Geometry: final body of the model. Coordinates: model frame, mm. Give positions to 0.01 mm unless a question says otherwise; leave off trailing zeros. Write each loop counter-clockwise with the first axis right and the second up, starting at its lowest first coordinate (ties: lowest second). Pieces come first, ordered by that corner, then holes. Notation, with made-up numbers: M 87,-10.5 L 121,-10.5 A24 ccw 121,28.5 Z; hole C 4,-19 d6. An arc over 180 degrees is marked long. Use a Markdown table: item, result. Add a question column.
(1) Cut plane C-C (x = 26.6). State how many separate pieces and enclosed holes the cut face has, plus the area to 3 significant figures.
(2) Pin query (flat end, axial travel): pin 1 Ø5 at (y, z) = (1, -15.5) entering from -X; pin 2 Ø12 at (x, z) = (-31, 3.5) entering from +Y; pin 3 Ø3.5 at (x, z) = (4.2, 10.4) entering from -Y. Return the tip coordinate at first contact, or that it passes through.
(3) Cut plane B-B (z = -17.5). Output: boundary loops of the cut face in (x, y), plus the area to 3 significant figures.
(4) Cut plane A-A (x = -168). Output: boundary loops of the cut face in (y, z), plus the area to 3 significant figures.
(5) Material intervals for L1, parallel to Y at x = -2, z = -4.5; L2, parallel to Z at x = -153, y = 3.5, sorted ascending.
```python
from build123d import *

# Parameters (mm, degrees)
SKETCH1_R           = 3
BOSS_EXTRUDE2_DEPTH = 5
SKETCH2_R           = 1.1
BOSS_EXTRUDE3_DEPTH = 5
FILLET1_R           = 1
CUT_EXTRUDE1_DEPTH  = 3


with BuildPart() as part:
    # Sketch1 → Boss-Extrude2 (new body)
    with BuildSketch(Plane(origin=(0, 0, 0), x_dir=(1, 0, 0), z_dir=(0, 1, 0))):
        Polygon((-35, 40), (35, 40), (35, -40), (-35, -40), (-172, -40), (-172, -34), (-172, 12), (-164, 12), (-164, -34), (-35, -34), align=None)
        with Locations((-18.2, 34.4)):
            Circle(SKETCH1_R, mode=Mode.SUBTRACT)
        with Locations((-7, 34.4)):
            Circle(SKETCH1_R, mode=Mode.SUBTRACT)
        with Locations((4.2, 34.4)):
            Circle(SKETCH1_R, mode=Mode.SUBTRACT)
        with Locations((15.4, 34.4)):
            Circle(SKETCH1_R, mode=Mode.SUBTRACT)
        with Locations((26.6, 34.4)):
            Circle(SKETCH1_R, mode=Mode.SUBTRACT)
        with Locations((-18.2, 23.2)):
            Circle(SKETCH1_R, mode=Mode.SUBTRACT)
        with Locations((-7, 23.2)):
            Circle(SKETCH1_R, mode=Mode.SUBTRACT)
        with Locations((4.2, 23.2)):
            Circle(SKETCH1_R, mode=Mode.SUBTRACT)
        with Locations((15.4, 23.2)):
            Circle(SKETCH1_R, mode=Mode.SUBTRACT)
        with Locations((26.6, 23.2)):
            Circle(SKETCH1_R, mode=Mode.SUBTRACT)
        with Locations((-18.2, 12)):
            Circle(SKETCH1_R, mode=Mode.SUBTRACT)
        with Locations((-7, 12)):
            Circle(SKETCH1_R, mode=Mode.SUBTRACT)
        with Locations((4.2, 12)):
            Circle(SKETCH1_R, mode=Mode.SUBTRACT)
        with Locations((15.4, 12)):
            Circle(SKETCH1_R, mode=Mode.SUBTRACT)
        with Locations((26.6, 12)):
            Circle(SKETCH1_R, mode=Mode.SUBTRACT)
        with Locations((-18.2, 0.8)):
            Circle(SKETCH1_R, mode=Mode.SUBTRACT)
        with Locations((-7, 0.8)):
            Circle(SKETCH1_R, mode=Mode.SUBTRACT)
        with Locations((4.2, 0.8)):
            Circle(SKETCH1_R, mode=Mode.SUBTRACT)
        with Locations((15.4, 0.8)):
            Circle(SKETCH1_R, mode=Mode.SUBTRACT)
        with Locations((26.6, 0.8)):
            Circle(SKETCH1_R, mode=Mode.SUBTRACT)
        with Locations((-18.2, -10.4)):
            Circle(SKETCH1_R, mode=Mode.SUBTRACT)
        with Locations((-7, -10.4)):
            Circle(SKETCH1_R, mode=Mode.SUBTRACT)
        with Locations((4.2, -10.4)):
            Circle(SKETCH1_R, mode=Mode.SUBTRACT)
        with Locations((15.4, -10.4)):
            Circle(SKETCH1_R, mode=Mode.SUBTRACT)
        with Locations((26.6, -10.4)):
            Circle(SKETCH1_R, mode=Mode.SUBTRACT)
        with Locations((-18.2, -21.6)):
            Circle(SKETCH1_R, mode=Mode.SUBTRACT)
        with Locations((-7, -21.6)):
            Circle(SKETCH1_R, mode=Mode.SUBTRACT)
        with Locations((4.2, -21.6)):
            Circle(SKETCH1_R, mode=Mode.SUBTRACT)
        with Locations((15.4, -21.6)):
            Circle(SKETCH1_R, mode=Mode.SUBTRACT)
        with Locations((26.6, -21.6)):
            Circle(SKETCH1_R, mode=Mode.SUBTRACT)
        with Locations((-7, -32.8)):
            Circle(SKETCH1_R, mode=Mode.SUBTRACT)
        with Locations((4.2, -32.8)):
            Circle(SKETCH1_R, mode=Mode.SUBTRACT)
        with Locations((15.4, -32.8)):
            Circle(SKETCH1_R, mode=Mode.SUBTRACT)
        with Locations((26.6, -32.8)):
            Circle(SKETCH1_R, mode=Mode.SUBTRACT)
        with Locations((-168, 4.718835642)):
            Circle(SKETCH1_R, mode=Mode.SUBTRACT)
        with Locations((-168, -28.604223743)):
            Circle(SKETCH1_R, mode=Mode.SUBTRACT)
        with BuildLine():
            Line((-26.219397272, 34.096793065), (-26.219397272, -34.303206935))
            ThreePointArc((-26.219397272, -34.303206935), (-27.819397272, -35.903206935), (-29.419397272, -34.303206935))
            Line((-29.419397272, -34.303206935), (-29.419397272, 34.096793065))
            ThreePointArc((-29.419397272, 34.096793065), (-27.819397272, 35.696793065), (-26.219397272, 34.096793065))
        make_face(mode=Mode.SUBTRACT)
    extrude(amount=BOSS_EXTRUDE2_DEPTH)

    # Sketch2 → Boss-Extrude3 (add)
    with BuildSketch(Plane(origin=(0, 5, 0), x_dir=(1, 0, 0), z_dir=(0, 1, 0))):
        with Locations((33, -30)):
            Circle(SKETCH2_R)
        with Locations((-15.999841725, -30.124542974)):
            Circle(SKETCH2_R)
        with Locations((-15.999841725, 28)):
            Circle(SKETCH2_R)
        with Locations((33, 28)):
            Circle(SKETCH2_R)
    extrude(amount=BOSS_EXTRUDE3_DEPTH)

    # Fillet1
    fillet1_edges = [part.edges().sort_by_distance(p)[0] for p in [
        (35, 2.5, 40),
        (-172, 2.5, 40),
        (-172, 2.5, -12),
        (-164, 2.5, -12),
        (-164, 2.5, 34),
        (-35, 2.5, 34),
        (-35, 2.5, -40),
        (35, 2.5, -40),
    ]]
    fillet(fillet1_edges, radius=FILLET1_R)

    # Sketch5 → Cut-Extrude1 (cut)
    with BuildSketch(Plane.XZ):
        with BuildLine():
            Line((-25.069397272, 34.303206935), (-25.069397272, -33.841459302))
            ThreePointArc((-25.069397272, -33.841459302), (-27.819397272, -36.591459302), (-30.569397272, -33.841459302))
            Line((-30.569397272, -33.841459302), (-30.569397272, 34.303206935))
            ThreePointArc((-30.569397272, 34.303206935), (-27.819397272, 37.053206935), (-25.069397272, 34.303206935))
        make_face()
    extrude(amount=-CUT_EXTRUDE1_DEPTH, mode=Mode.SUBTRACT)


solid = part.part
```
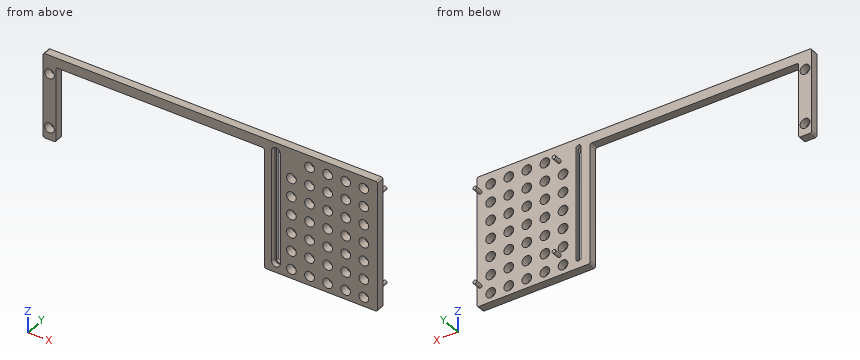
Answer list:
| question | item | result |
|---|---|---|
| 1 | separate pieces | 8 |
| 1 | enclosed holes | 0 |
| 1 | area | 190 mm² |
| 2 | pin 1 | x = -35 |
| 2 | pin 2 | y = 5 |
| 2 | pin 3 | through |
| 3 | outline | M -35,0 L -30.57,0 L -30.57,3 L -29.42,3 L -29.42,5 L -35,5 Z; M -26.22,3 L -25.07,3 L -25.07,0 L 35,0 L 35,5 L -26.22,5 Z |
| 3 | area | 327 mm² |
| 4 | outline | M 0,-12 L 5,-12 L 5,-7.72 L 0,-7.72 Z; M 0,-1.72 L 5,-1.72 L 5,25.6 L 0,25.6 Z; M 0,31.6 L 5,31.6 L 5,40 L 0,40 Z |
| 4 | area | 200 mm² |
| 5 | L1 | 0 to 5 |
| 5 | L2 | 34 to 40 |
